from build123d import *

# Parameters (mm, degrees)
SKETCH_1_R          = 5.3
EXTRUDE_1_DEPTH     = 0.8
EXTRUDE_2_DEPTH     = 2.2
CUT_EXTRUDE_1_DEPTH = 0.5
SKETCH_5_W          = 1.290577963
SKETCH_5_H          = 8.1
EXTRUDE_5_DEPTH     = 1.4
SKETCH_4_W          = 2.5
SKETCH_4_H          = 2.5
EXTRUDE_4_DEPTH     = 0.2


with BuildPart() as part:
    # Эскиз1 → Бобышка-Вытянуть1 (new body)
    with BuildSketch(Plane.XY):
        Circle(SKETCH_1_R)
    extrude(amount=EXTRUDE_1_DEPTH)

    # Эскиз2 → Бобышка-Вытянуть2 (add)
    with BuildSketch(Plane.XY.offset(0.8)):
        with BuildLine():
            Line((3, -7), (-3, -7))
            ThreePointArc((-3, -7), (-10, 0), (-3, 7))
            Line((-3, 7), (3, 7))
            ThreePointArc((3, 7), (10, 0), (3, -7))
        make_face()
    extrude(amount=EXTRUDE_2_DEPTH)

    # Эскиз3 → Вырез-Вытянуть1 (cut)
    with BuildSketch(Plane.XY.offset(3)):
        with BuildLine():
            Line((-3, 5.25), (3, 5.25))
            ThreePointArc((3, 5.25), (8.25, 0), (3, -5.25))
            Line((3, -5.25), (-3, -5.25))
            ThreePointArc((-3, -5.25), (-8.25, 0), (-3, 5.25))
        make_face()
    extrude(amount=-CUT_EXTRUDE_1_DEPTH, mode=Mode.SUBTRACT)

    # Эскиз5 → Бобышка-Вытянуть5 (add)
    with BuildSketch(Plane(origin=(0, 0, 0.8), x_dir=(-1, 0, 0), z_dir=(0, 0, -1))):
        with Locations((9.354711019, 0)):
            Rectangle(SKETCH_5_W, SKETCH_5_H)
    extrude(amount=-EXTRUDE_5_DEPTH)

    # Эскиз4 → Бобышка-Вытянуть4 (add)
    with BuildSketch(Plane(origin=(0, 0, 0.8), x_dir=(-1, 0, 0), z_dir=(0, 0, -1))):
        with Locations((8.45, 2.5)):
            Rectangle(SKETCH_4_W, SKETCH_4_H)
        with Locations((8.45, -2.5)):
            Rectangle(SKETCH_4_W, SKETCH_4_H)
    extrude(amount=EXTRUDE_4_DEPTH)


solid = part.part
Source: CAD feature listing. Evaluate the final solid. Frame: model axes, mm. A direction names the side the tool comes from. Give positions to 0.01 mm unless a question says otherwise; leave off trailing zeros. Order: outer loops, then holes, each group sorted by start corner. A loop starts at its lowest first (then second) coordinate and runs counter-clockwise, first axis right, second up. Notation, with made-up numbers: (14, 17.25) -> (29, 17.25) arc R14 cw to (29, 27.25) -> close; hole circle Ø5 at (34.5, 71). An arc over 180 degrees is marked (long way). Write item = value, one per line.
Q1. Pull-direction query (Y, two-part tool) for faces 6 (the face through (0, -7, 2)), 7 (the face through (0, 0, 0)), 8 (the face through (0, 7, 2)), 9 (the face through (0, 0, 2.5)); classes: released by +Y, released by -Y, zero draft, split by the parting line, or undercut.
Data:
face_6 = released by -Y
face_7 = zero draft
face_8 = released by +Y
face_9 = undercut
Q2. Cut plane D-D, the plane z = 1.4. Output: boundary loops of the cut face in (x, y).
Data:
outline = (-10, -4.05) -> (-8.71, -4.05) arc R7 ccw to (-3, -7) -> (3, -7) arc R7 ccw to (3, 7) -> (-3, 7) arc R7 ccw to (-8.71, 4.05) -> (-10, 4.05) -> close
Q3. Pin query (flat end, axial travel): pin 1 (1 mm diameter, centred on x = -9.5, z = 1.5, fed in from +Y); pin 2 (1.2 mm diameter, centred on x = -8, y = -3, fed in from -Z); pin 3 (4 mm diameter, centred on x = -1.5, y = 2.5, fed in from +Z). Return the tip coordinate at first contact, or that it passes through.
Data:
pin_1 = 4.05
pin_2 = 0.6
pin_3 = 2.5
Q4. Cut plane B-B, the plane z = 2.75. Output: boundary loops of the cut face in (x, y).
Data:
outline = (-3, -7) -> (3, -7) arc R7 ccw to (3, 7) -> (-3, 7) arc R7 ccw to start; hole (-3, -5.25) -> (3, -5.25) arc R5.25 ccw to (3, 5.25) -> (-3, 5.25) arc R5.25 ccw to start
Q5. Cut plane A-A, the plane x = 0. Output: boundary loops of the cut face in (y, z).
Data:
outline = (-7, 0.8) -> (-5.3, 0.8) -> (-5.3, 0) -> (5.3, 0) -> (5.3, 0.8) -> (7, 0.8) -> (7, 3) -> (5.25, 3) -> (5.25, 2.5) -> (-5.25, 2.5) -> (-5.25, 3) -> (-7, 3) -> close
Q6. Cut plane C-C, the plane y = 2.75. Output: boundary loops of the cut face in (x, z), and give its area (3 significant figures).
Data:
outline = (-10, 0.8) -> (-9.7, 0.8) -> (-9.7, 0.6) -> (-7.2, 0.6) -> (-7.2, 0.8) -> (-4.53, 0.8) -> (-4.53, 0) -> (4.53, 0) -> (4.53, 0.8) -> (9.44, 0.8) -> (9.44, 3) -> (7.47, 3) -> (7.47, 2.5) -> (-7.47, 2.5) -> (-7.47, 3) -> (-9.44, 3) -> (-9.44, 2.2) -> (-10, 2.2) -> close
area = 42.6 mm^2
Q7. Set-up query: faces 1 (the face through (4.896, -2.03, 0.394)), 2 (the face through (-9, -4.05, 1)), 3 (the face through (8.25, 0.12, 2.75)), 4 (the face through (-8, -2, 0.6)), 5 (the face through (-9.6, 2.9, 2.2)). Return all of +Z, -Z, +X, -X, +Y, -Y with unobstructed straight access to the full face (end or side cutting, diameter ignored); none if empty.
Data:
face_1 = -Z
face_2 = +Z, -Z, -X, -Y
face_3 = +Z
face_4 = -Z, -X, +Y, -Y
face_5 = +Z, -X, +Y
Q8. Material intervals for line 1 (Y direction, x = -1, z = 2.6); line 2 (Z direction, x = -7, y = -5.25); line 3 (Z direction, x = -4.5, y = 3), sorted ascending. Write a range as from..to.
Data:
line_1 = -7..-5.25, 5.25..7
line_2 = 0.8..3
line_3 = 0.8..2.5
